```python
from build123d import *

# Parameters (mm, degrees)
F0_W     = 100
F0_H     = 100
F1_DEPTH = 100
F3_DEPTH = 100
F5_DEPTH = 100
F7_DEPTH = 100


with BuildPart() as f1:
    # F0 (on Front) → F1 (new body)
    with BuildSketch(Plane.XZ):
        with Locations((6.997038, -9.774505)):
            Rectangle(F0_W, F0_H)
    extrude(amount=F1_DEPTH)

    # F2 (on face) → F3 (cut)
    with BuildSketch(Plane.XY.offset(40.225495)):
        Polygon((56.997038, 0), (-43.002962, -100), (56.997038, -100), align=None)
    extrude(amount=-F3_DEPTH, mode=Mode.SUBTRACT)

    # F4 (on face) → F5 (cut)
    with BuildSketch(Plane(origin=(-43.002962, 0, 0), x_dir=(0, -1, 0), z_dir=(-1, 0, 0))):
        Polygon((100, -59.774505), (100, 40.225495), (0, -59.774505), align=None)
    extrude(amount=-F5_DEPTH, mode=Mode.SUBTRACT)

    # F6 (on face) → F7 (cut)
    with BuildSketch(Plane(origin=(0, 0, 0), x_dir=(-1, 0, 0), z_dir=(0, 1, 0))):
        Polygon((-56.997038, -59.774505), (43.002962, -59.774505), (-56.997038, 40.225495), align=None)
    extrude(amount=-F7_DEPTH, mode=Mode.SUBTRACT)


solid = f1.part
```
The listing builds one solid part. Answer for the finished solid, in the listing's coordinates (mm). Round coordinates to 2 decimals unless told otherwise and drop trailing zeros. Write each loop counter-clockwise with the first axis right and the second up, starting at its lowest first coordinate (ties: lowest second). Pieces come first, ordered by that corner, then holes. Notation, with made-up numbers: (25.5, 83) -> (33.5, 83) arc R29 cw to (33.5, 116) -> close; hole circle Ø11 at (39, -6). An arc over 180 degrees is marked (long way). Answer as a JSON object with one key per item and string values. Group by question number.
Q1. Section B-B (x = -19.5) is taken. Write down the section's boundary in (y, z).
Q2. Section D-D (y = -69.5) is taken. Write down the section's boundary in (x, z).
Q3. Each of these flat-tipped pins is pushed along its axis until it touches: pin 1 Ø2 at (y, z) = (-82.5, 28) entering from +X; pin 2 Ø3 at (x, z) = (10.5, 7) entering from -Y; pin 3 Ø2 at (x, z) = (0.5, 11) entering from -Y. Where does it stop, or does it pass through?
Q4. Section A-A (y = -11.5) is taken. Write down the section's boundary in (x, z).
Q5. Straight lines are drawn through the part: line 1 along Y through (x, z) = (-3, 35.5); line 2 along X through (y, z) = (-37, 10.5); line 3 along X through (y, z) = (-74, 32.5). For each, find the intervals that lie inside material, in ascending order.
Q6. Section C-C (z = -30) is taken. Write down the section's boundary in (x, y).
Check values:
{
 "1": {"outline": "(-76.5, 16.72) -> (-23.5, -36.27) -> (0, -36.27) -> (0, 40.23) -> (-76.5, 40.23) -> close"},
 "2": {"outline": "(-43, 9.73) -> (-12.5, 9.73) -> (-12.5, 40.23) -> (-43, 40.23) -> close"},
 "3": {"pin 1": "x = -24.5", "pin 2": "y = -48", "pin 3": "y = -57.5"},
 "4": {"outline": "(-43, -48.27) -> (-31.5, -48.27) -> (45.5, 28.73) -> (45.5, 40.23) -> (-43, 40.23) -> close"},
 "5": {"line 1": "-60 to 0", "line 2": "-43 to 20", "line 3": "-43 to -17"},
 "6": {"outline": "(-43, -29.77) -> (-13.23, -29.77) -> (-13.23, 0) -> (-43, 0) -> close"}
}
